CAD build for the part. Positions are in the model's coordinates, mm. A direction names the side the tool comes from. Round coordinates to 2 decimals unless told otherwise and drop trailing zeros. Loops run counter-clockwise (first coordinate to the right, second up) from the corner with the lowest first, then second, coordinate; pieces in that order, holes last.
```python
from build123d import *

# Parameters (mm, degrees)
SKETCH006_R  = 2.3
PAD006_DEPTH = 100
SKETCH005_W  = 216
SKETCH005_H  = 20
PAD005_DEPTH = 4
SKETCH004_R  = 4
PAD004_DEPTH = 50
SKETCH003_R  = 1.5
PAD003_DEPTH = 100
SKETCH002_R  = 5
PAD002_DEPTH = 30
SKETCH001_W  = 210.6
SKETCH001_H  = 127
PAD001_DEPTH = 33
SKETCH_W     = 216
SKETCH_H     = 130
PAD_DEPTH    = 36


with BuildPart() as sensor_head_mount_holes:
    # Sketch006 → Pad006 (new body)
    with BuildSketch(Plane.XY):
        with Locations((18, 42)):
            Circle(SKETCH006_R)
        with Locations((198, 42)):
            Circle(SKETCH006_R)
        with Locations((18, 92)):
            Circle(SKETCH006_R)
        with Locations((198, 92)):
            Circle(SKETCH006_R)
    extrude(amount=PAD006_DEPTH)


with BuildPart() as crossbeams:
    # Sketch005 → Pad005 (new body)
    with BuildSketch(Plane.XY.offset(29)):
        with Locations((108, 92)):
            Rectangle(SKETCH005_W, SKETCH005_H)
        with Locations((108, 42)):
            Rectangle(SKETCH005_W, SKETCH005_H)
    extrude(amount=PAD005_DEPTH)


with BuildPart() as screw_recesses:
    # Sketch004 → Pad004 (new body)
    with BuildSketch(Plane.XY.offset(8)):
        with Locations((7, 123)):
            Circle(SKETCH004_R)
        with Locations((7, 16)):
            Circle(SKETCH004_R)
        with Locations((209, 123)):
            Circle(SKETCH004_R)
        with Locations((209, 16)):
            Circle(SKETCH004_R)
    extrude(amount=PAD004_DEPTH)


with BuildPart() as screw_holes:
    # Sketch003 → Pad003 (new body)
    with BuildSketch(Plane.XY):
        with Locations((7, 123)):
            Circle(SKETCH003_R)
        with Locations((7, 16)):
            Circle(SKETCH003_R)
        with Locations((209, 123)):
            Circle(SKETCH003_R)
        with Locations((209, 16)):
            Circle(SKETCH003_R)
    extrude(amount=PAD003_DEPTH)


with BuildPart() as pylons:
    # Sketch002 → Pad002 (new body)
    with BuildSketch(Plane.XY.offset(3)):
        with Locations((7, 123)):
            Circle(SKETCH002_R)
        with Locations((7, 16)):
            Circle(SKETCH002_R)
        with Locations((209, 123)):
            Circle(SKETCH002_R)
        with Locations((209, 16)):
            Circle(SKETCH002_R)
    extrude(amount=PAD002_DEPTH)


with BuildPart() as interior_hole:
    # Sketch001 → Pad001 (new body)
    with BuildSketch(Plane.XY):
        with Locations((108, 63.5)):
            Rectangle(SKETCH001_W, SKETCH001_H)
    extrude(amount=PAD001_DEPTH)


with BuildPart() as cut003:
    # Sketch → Pad (new body)
    with BuildSketch(Plane.XY):
        with Locations((108, 65)):
            Rectangle(SKETCH_W, SKETCH_H)
    extrude(amount=PAD_DEPTH)

    # Cut: cut Interior Hole
    add(interior_hole.part, mode=Mode.SUBTRACT)

    # Fusion: union Pylons
    add(pylons.part)

    # Cut001: cut Screw Holes
    add(screw_holes.part, mode=Mode.SUBTRACT)

    # Cut002: cut Screw Recesses
    add(screw_recesses.part, mode=Mode.SUBTRACT)

    # Fusion001: union Crossbeams
    add(crossbeams.part)

    # Cut003: cut Sensor Head Mount Holes
    add(sensor_head_mount_holes.part, mode=Mode.SUBTRACT)


solid = cut003.part
```
Item 1: Cut at A-A, the plane y = 92. Give the cut face in (x, z), plus the area to 3 significant figures.
Answers follow:
outline: (0, 0) - (2.7, 0) - (2.7, 29) - (15.7, 29) - (15.7, 36) - (0, 36) - close; (20.3, 29) - (195.7, 29) - (195.7, 36) - (20.3, 36) - close; (200.3, 29) - (213.3, 29) - (213.3, 0) - (216, 0) - (216, 36) - (200.3, 36) - close
area: 1,600 mm2
Item 2: Flat gauge pins, fed straight in: P1, Ø7, axis at x = 209, y = 16, coming from the -Z side; P2, Ø1.5, axis at x = 124.5, z = 15.5, coming from the -Y side; P3, Ø2.5, axis at x = 209, y = 16, coming from the -Z side; P4, Ø2.5, axis at x = 207.5, y = 16.5, coming from the +Z side. Where does each tip first touch, or does it go through?
Answers follow:
P1: stops at z = 3
P2: stops at y = 127
P3: passes through
P4: stops at z = 8
Item 3: Two-plate mould, pull along Y, no slides. Class faces 5 (the flat face through (107, 102, 31)), 6 (the flat face through (106, 66, 36)), 7 (the flat face through (107, 0, 35)): released by +Y, released by -Y, zero draft, split by the parting line, or undercut.
Answers follow:
face 5: undercut
face 6: zero draft
face 7: released by -Y
Item 4: Cut at C-C, the plane z = 22. Give the cut face in (x, y).
Answers follow:
outline: (0, 0) - (2.7, 0) - (2.7, 13.45) arc R5 ccw (long way) to (2.7, 18.55) - (2.7, 120.45) arc R5 ccw (long way) to (10, 127) - (206, 127) arc R5 ccw (long way) to (213.3, 120.45) - (213.3, 18.55) arc R5 ccw (long way) to (213.3, 13.45) - (213.3, 0) - (216, 0) - (216, 130) - (0, 130) - close; hole (2.7, 125.55) arc R5 cw to (4, 127) - (2.7, 127) - close; hole circle Ø8 at (7, 16); hole circle Ø8 at (7, 123); hole circle Ø8 at (209, 16); hole circle Ø8 at (209, 123); hole (212, 127) arc R5 cw to (213.3, 125.55) - (213.3, 127) - close
Item 5: 3-axis set-ups, long thin cutter, end or side, ignore diameter. For faces 1 (the cylindrical face through (197.501, 89.755, 32.451)), 2 (the flat face through (8.3, 121.6, 3)), 3 (the cylindrical face through (6.479, 126.966, 21.804)), 4 (the flat face through (107, 52, 31)): which of +Z, -Z, +X, -X, +Y, -Y reach the whole face in a straight line?
Answers follow:
face 1: +Z, -Z
face 2: -Z, -Y
face 3: +Z
face 4: -Z
Item 6: Cut at B-B, the plane x = 198. Give the cut face in (y, z), plus the area to 3 significant figures.
Answers follow:
outline: (0, 33) - (32, 33) - (32, 29) - (39.7, 29) - (39.7, 36) - (0, 36) - close; (44.3, 29) - (52, 29) - (52, 33) - (82, 33) - (82, 29) - (89.7, 29) - (89.7, 36) - (44.3, 36) - close; (94.3, 29) - (102, 29) - (102, 33) - (127, 33) - (127, 0) - (130, 0) - (130, 36) - (94.3, 36) - close
area: 585 mm2
Item 7: Probe line 1 (Y direction, x = 209, z = 18); line 2 (X direction, y = 123, z = 4.45); line 3 (Y direction, x = 209, z = 29.5). List the from-to ranges inside material, lowest first.
Answers follow:
line 1: y = 11 to 12, 20 to 21, 118 to 119, 127 to 130
line 2: x = 0 to 5.5, 8.5 to 12, 204 to 207.5, 210.5 to 216
line 3: y = 11 to 12, 20 to 21, 32 to 52, 82 to 102, 118 to 119, 127 to 130
Item 8: Cut at D-D, the plane x = 146.5. Give the cut face in (y, z).
Answers follow:
outline: (0, 33) - (32, 33) - (32, 29) - (52, 29) - (52, 33) - (82, 33) - (82, 29) - (102, 29) - (102, 33) - (127, 33) - (127, 0) - (130, 0) - (130, 36) - (0, 36) - close
